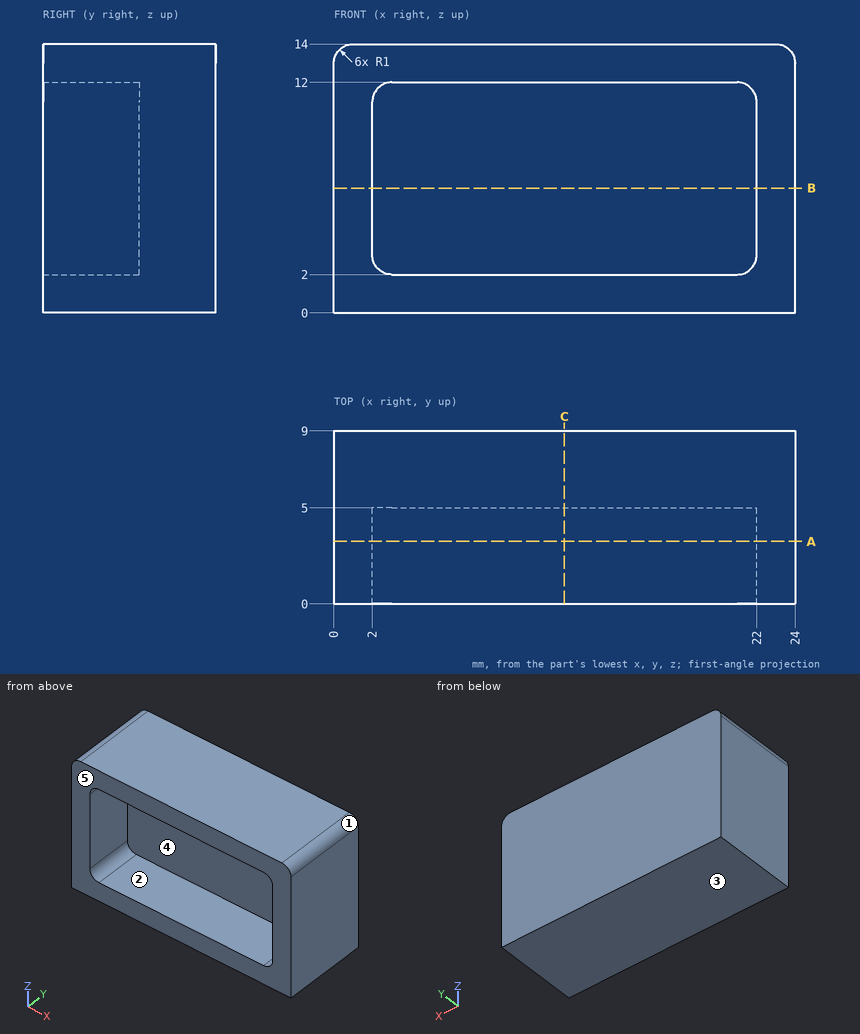
Geometry: see drawing. Coordinates: mm, zero at the bounding-box minimum. A direction names the side the tool comes from. Coordinates: 2 decimals unless noted, no trailing zeros. Order: outer loops, then holes, each group sorted by start corner. A loop starts at its lowest first (then second) coordinate and runs counter-clockwise, first axis right, second up. Notation, with made-up numbers: M 79.25,16.5 L 126.25,16.5 A32 ccw 126.25,55.5 Z; hole C -10,58.5 d5. An arc over 180 degrees is marked long. Answer in a Markdown table with one row per item. Add a question column.
Q1. Mould query, pull axis Z, two halves, no side actions, for the marked faces 3, 4 and 5. Classes: released by +Z, released by -Z, zero draft, split by the parting line, or undercut.
Q2. Contact query for a flat-ended pin moving along its axis: P1, Ø3, axis at x = 10.5, z = 7.5, coming from the -Y side. Output: stop coordinate, or through.
Q3. Section query B-B on z = 6.5. Return the cut outline in (x, y), and give its area (3 significant figures).
Q4. Section query C-C on x = 12. Return the cut outline in (y, z).
Q5. Section query A-A on y = 3.25. Return the cut outline in (x, z), and give its area (3 significant figures).
Q6. Reachability of the marked faces 1 and 2 from +Z, -Z, +X, -X, +Y, -Y: full face, straight path, thin tool, end or side. Return the list, or none.
Q7. Line query: L1, parallel to X at y = 3.5, z = 6; L2, parallel to Z at x = 16, y = 1.5; L3, parallel to Y at x = 13.5, z = 3.25. Output: solid intervals per line, ascending.
Completed:
| question | item | result |
|---|---|---|
| 1 | face 3 | released by -Z |
| 1 | face 4 | undercut |
| 1 | face 5 | zero draft |
| 2 | P1 | stops at y = 5 |
| 3 | outline | M 0,0 L 2,0 L 2,5 L 22,5 L 22,0 L 24,0 L 24,9 L 0,9 Z |
| 3 | area | 116 mm2 |
| 4 | outline | M 0,0 L 9,0 L 9,14 L 0,14 L 0,12 L 5,12 L 5,2 L 0,2 Z |
| 5 | outline | M 0,0 L 24,0 L 24,13 A1 ccw 23,14 L 1,14 A1 ccw 0,13 Z; hole M 2,3 A1 ccw 3,2 L 21,2 A1 ccw 22,3 L 22,11 A1 ccw 21,12 L 3,12 A1 ccw 2,11 Z |
| 5 | area | 136 mm2 |
| 6 | face 1 | +Z, +X, +Y, -Y |
| 6 | face 2 | -Y |
| 7 | L1 | x = 0 to 2, 22 to 24 |
| 7 | L2 | z = 0 to 2, 12 to 14 |
| 7 | L3 | y = 5 to 9 |
